Part model, mm, in its own coordinate system. Coordinates: 2 decimals unless noted, no trailing zeros. Loops run counter-clockwise (first coordinate to the right, second up) from the corner with the lowest first, then second, coordinate; pieces in that order, holes last. Notation, with made-up numbers: (15, 42) -> (63, 42) arc R26 cw to (63, 72) -> close; hole circle Ø3 at (39.5, 83.5). An arc over 180 degrees is marked (long way). Use one line per item in the form item = value. Start each with the question number.
(1) Drill centre lines: L1, parallel to Y at x = -3, z = 1.3; L2, parallel to Y at x = 11, z = 2.6; L3, parallel to Y at x = 5.5, z = 4.4. Where is each one in solid material? Low to high. Write a range as [from, to].
(2) Band-saw the part on D-D on x = 4.5. Give the cut face in (y, z).
(3) Band-saw the part on B-B on y = 107. Give the cut face in (x, z).
(4) Band-saw the part on C-C on z = 1.5. Give the cut face in (x, y).
(5) Pin check, flat tips, straight feed: P1, Ø2.5, axis at y = 121, z = 3.5, coming from the -X side; P2, Ø2, axis at y = 46, z = 2.5, coming from the -X side. Stop position of each tip, or through.
(6) Band-saw the part on A-A on x = 19. Give the cut face in (y, z), then the cut area to 3 significant figures.
```python
from build123d import *

# Parameters (mm, degrees)
F1_DEPTH = 5
F2_R     = 7.9883
F3_DEPTH = 25.4
F6_DEPTH = 25.4
F7_R     = 6.35


with BuildPart() as f1:
    # F0 (on Top) → F1 (new body)
    with BuildSketch(Plane.XY):
        with BuildLine():
            Line((1.470284, 287.84881), (0, 0))
            Line((0, 0), (36.98494, 0))
            Line((36.98494, 0), (58.59907, 80.73898))
            Line((58.59907, 80.73898), (58.59907, 182.05958))
            Line((58.59907, 182.05958), (50.6857, 315.67628))
            Line((50.6857, 315.67628), (34.044278, 314.690702))
            ThreePointArc((34.044278, 314.690702), (22.258545, 295.807244), (1.470284, 287.84881))
        make_face()
        with BuildLine():
            Line((-36.98301, 0.377816), (0, 0))
            Line((0, 0), (1.470284, 287.84881))
            ThreePointArc((1.470284, 287.84881), (-19.235594, 296.019189), (-30.82781, 315.022057))
            Line((-30.82781, 315.022057), (-47.458296, 316.177583))
            Line((-47.458296, 316.177583), (-56.736201, 182.648693))
            Line((-56.736201, 182.648693), (-57.771231, 81.33338))
            Line((-57.771231, 81.33338), (-36.98301, 0.377816))
        make_face()
    extrude(amount=F1_DEPTH)

    # F2 (on face) → F3 (cut)
    with BuildSketch(Plane.XY.offset(5)):
        with Locations((0, 249.86996)):
            Circle(F2_R)
        with Locations((0, 26.06802)):
            Circle(F2_R)
    extrude(amount=-F3_DEPTH, mode=Mode.SUBTRACT)

    # F5 (on face) → F6 (cut)
    with BuildSketch(Plane.XY.offset(5)):
        with BuildLine():
            ThreePointArc((-29.24937, 96.96323), (-20.682428, 76.280802), (0, 67.71386))
            ThreePointArc((0, 67.71386), (20.682428, 76.280802), (29.24937, 96.96323))
            Line((29.24937, 96.96323), (29.24937, 152.81021))
            ThreePointArc((29.24937, 152.81021), (20.682428, 173.492638), (0, 182.05958))
            ThreePointArc((0, 182.05958), (-20.682428, 173.492638), (-29.24937, 152.81021))
            Line((-29.24937, 152.81021), (-29.24937, 96.96323))
        make_face()
    extrude(amount=-F6_DEPTH, mode=Mode.SUBTRACT)

    # F7
    f7_edges = [f1.edges().sort_by_distance(p)[0] for p in [
        (-36.98301, 0.377816, 2.5),
        (36.98494, 0, 2.5),
        (50.6857, 315.67628, 2.5),
        (34.044278, 314.690702, 2.5),
        (-30.82781, 315.022057, 2.5),
        (-47.458296, 316.177583, 2.5),
    ]]
    fillet(f7_edges, radius=F7_R)


solid = f1.part
```
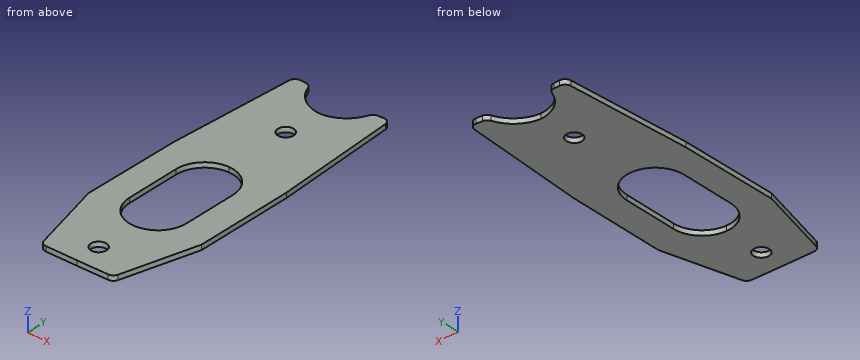
A:
q1.L1 = [0.03, 18.66], [33.47, 67.87], [181.91, 242.47], [257.27, 288.37]
q1.L2 = [0, 69.86], [179.91, 289.59]
q1.L3 = [0, 20.27], [31.86, 68.24], [181.54, 244.08], [255.66, 288.25]
q2.outline = (0, 0) -> (19.47, 0) -> (19.47, 5) -> (0, 5) -> close; (32.67, 0) -> (68.06, 0) -> (68.06, 5) -> (32.67, 5) -> close; (181.71, 0) -> (243.27, 0) -> (243.27, 5) -> (181.71, 5) -> close; (256.47, 0) -> (288.11, 0) -> (288.11, 5) -> (256.47, 5) -> close
q3.outline = (-57.51, 0) -> (-29.25, 0) -> (-29.25, 5) -> (-57.51, 5) -> close; (29.25, 0) -> (58.6, 0) -> (58.6, 5) -> (29.25, 5) -> close
q4.outline = (-57.77, 81.33) -> (-38.2, 5.1) arc R6.35 ccw to (-32.11, 0.33) -> (0, 0) -> (32.11, 0) arc R6.35 ccw to (38.25, 4.71) -> (58.6, 80.74) -> (58.6, 182.06) -> (51.06, 309.34) arc R6.35 ccw to (44.35, 315.3) -> (38.46, 314.95) arc R6.35 ccw to (32.87, 310.79) arc R35 cw to (1.47, 287.85) arc R35 cw to (-29.69, 311.11) arc R6.35 ccw to (-35.24, 315.33) -> (-41.12, 315.74) arc R6.35 ccw to (-47.9, 309.84) -> (-56.74, 182.65) -> close; hole (-29.25, 96.96) arc R29.25 ccw to (29.25, 96.96) -> (29.25, 152.81) arc R29.25 ccw to (-29.25, 152.81) -> close; hole circle Ø15.98 at (0, 26.07); hole circle Ø15.98 at (0, 249.87)
q5.P1 = -57.38
q5.P2 = -48.95
q6.outline = (0, 0) -> (74.73, 0) -> (74.73, 5) -> (0, 5) -> close; (175.05, 0) -> (293.42, 0) -> (293.42, 5) -> (175.05, 5) -> close
q6.area = 966 mm²
